Geometry check sheet. Reference: drawing and pictorial views, mm from the part's lowest x, y, z. A direction names the side the tool comes from. Give positions to 0.01 mm unless a question says otherwise; leave off trailing zeros. Loops run counter-clockwise (first coordinate to the right, second up) from the corner with the lowest first, then second, coordinate; pieces in that order, holes last. Notation, with made-up numbers: M -15.75,-18 L 43.25,-18 A20 cw 43.25,-4 Z; hole C 52.25,-39.5 d3. An arc over 180 degrees is marked long. Use CSV: the item, a comma, the result in double quotes.
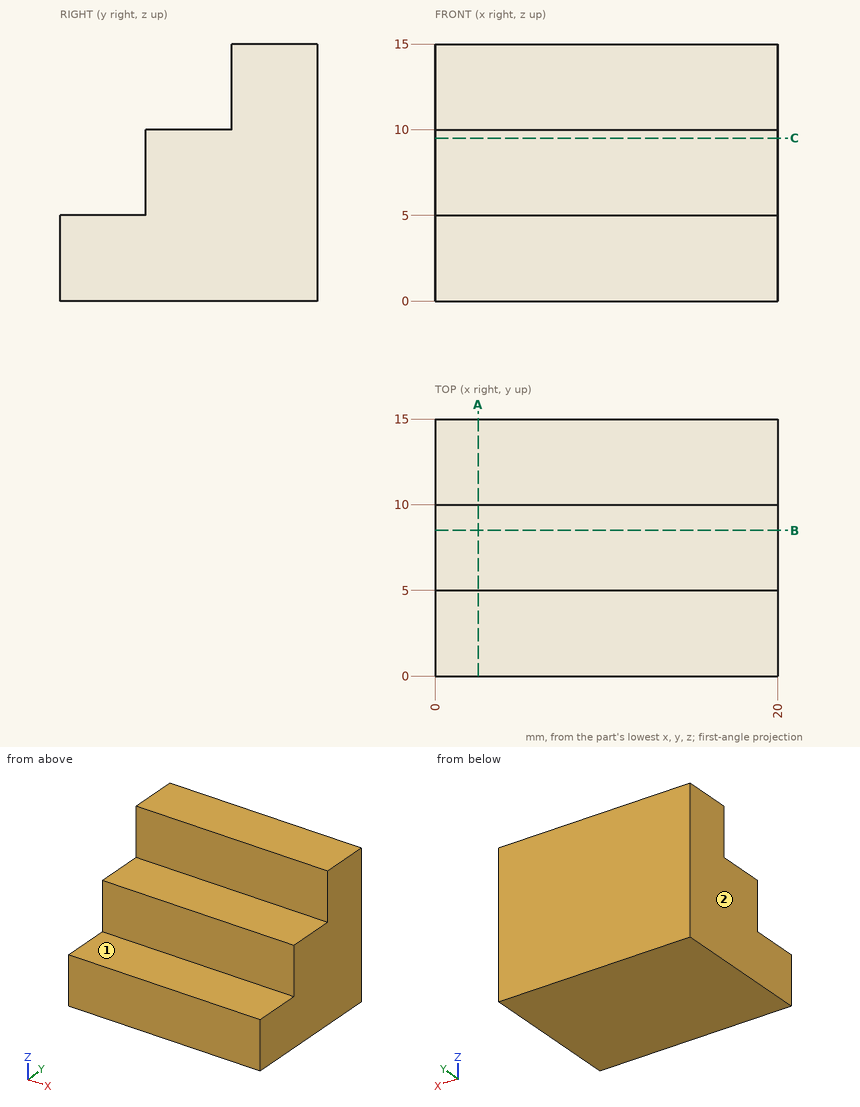
(1) Section check B-B on y = 8.5. Record the cut outline in (x, z).
Calculated:
outline,"M 0,0 L 20,0 L 20,10 L 0,10 Z"
(2) Section check A-A on x = 2.5. Record the cut outline in (y, z), plus the area to 3 significant figures.
Calculated:
outline,"M 0,0 L 15,0 L 15,15 L 10,15 L 10,10 L 5,10 L 5,5 L 0,5 Z"
area,"150 mm²"
(3) Scan lines: L1, parallel to Z at x = 12.5, y = 5.5; L2, parallel to Y at x = 15.5, z = 6; L3, parallel to Y at x = 12.75, z = 13.25. Record each from-to range of solid material in increasing order. Write a range as from..to.
Calculated:
L1,"z = 0..10"
L2,"y = 5..15"
L3,"y = 10..15"
(4) Section check C-C on z = 9.5. Record the cut outline in (x, y).
Calculated:
outline,"M 0,5 L 20,5 L 20,15 L 0,15 Z"
(5) Tool access check on the marked faces 1 and 2. Record the directions out of +Z, -Z, +X, -X, +Y, -Y that give a thin tool (end or side, any length) a straight path to the whole face; none if there is none.
Calculated:
face 1,"+Z, +X, -X, -Y"
face 2,"+Z, -Z, -X, +Y, -Y"
(6) Depth check by flat-ended pin: pin 1 Ø2.5 at (x, z) = (9, 11.5) entering from -Y; pin 2 Ø1.5 at (x, z) = (6, 7.5) entering from -Y; pin 3 Ø5.5 at (x, y) = (12.5, 2) entering from +Z. Enter the tip coordinate at first touch or a pass-through.
Calculated:
pin 1,"stops at y = 10"
pin 2,"stops at y = 5"
pin 3,"stops at z = 5"
